Job drawing, mm, ordinate dimensions from the low corner. One solid piece. Coordinates: 2 decimals unless noted, no trailing zeros. Loops run counter-clockwise (first coordinate to the right, second up) from the corner with the lowest first, then second, coordinate; pieces in that order, holes last. Notation, with made-up numbers: (-29.5, -19) - (20.5, -19) arc R29 cw to (20.5, 9) - close; hole circle Ø2 at (76, 85.5). An arc over 180 degrees is marked (long way). Use a Markdown table: item, result. Add a question column.
1. Band-saw the part on A-A, the plane z = 23.5. Give the cut face in (x, y) (1 decimal), plus the area to 3 significant figures.
2. Band-saw the part on C-C, the plane z = 47. Give the cut face in (x, y) (1 decimal).
3. Band-saw the part on B-B, the plane y = 2.45. Count the separate pieces of the cut face and the enclosed holes in it, plus the area to 3 significant figures.
4. Wall check: probe 1 along X at (y, z) = (1.45, 32) (1 decimal); probe 2 along X at (y, z) = (0.55, 47) (1 decimal); probe 3 along Z at (x, y) = (43, 0.5) (1 decimal). Give the ranges that are in metal, low to high. Write a range as [from, to].
5. Drop flat-ended pins along their axis: pin 1 (1 mm diameter, centred on y = 1.5, z = 40, fed in from +X) (1 decimal); pin 2 (1.6 mm diameter, centred on y = 1, z = 36, fed in from -X). Give the stop position or say it passes through.
6. Band-saw the part on D-D, the plane x = 32. Give the cut face in (y, z) (1 decimal).
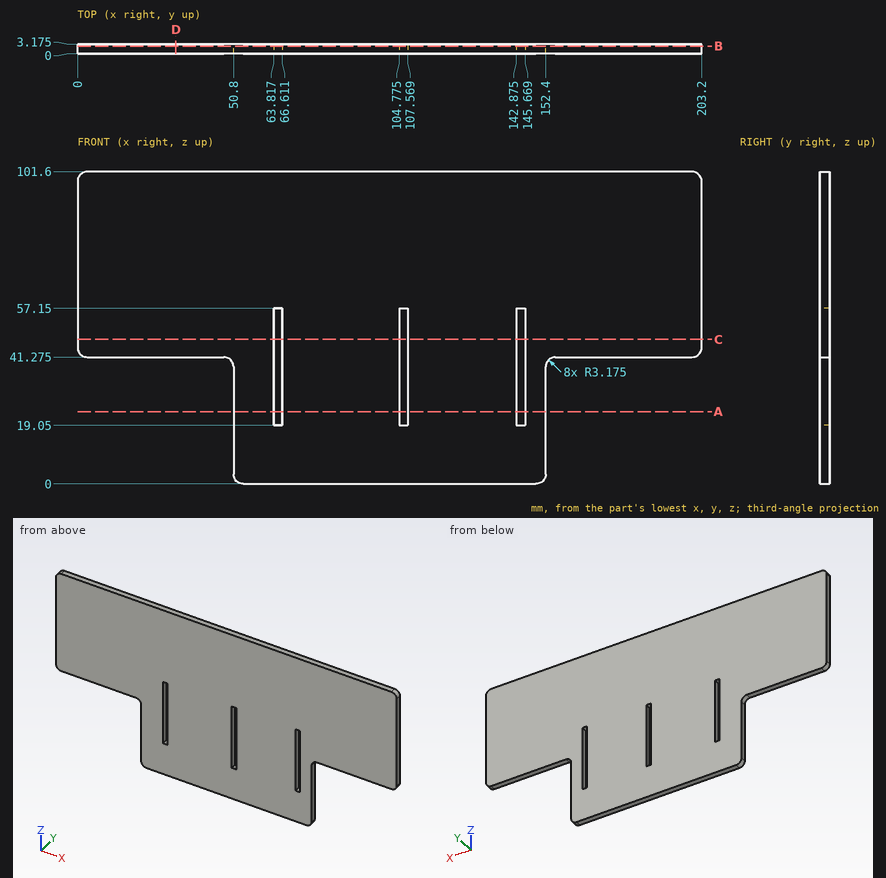
Geometry check:
| question | item | result |
|---|---|---|
| 1 | outline | (50.8, 0) - (63.8, 0) - (63.8, 3.2) - (50.8, 3.2) - close; (66.6, 0) - (104.8, 0) - (104.8, 3.2) - (66.6, 3.2) - close; (107.6, 0) - (142.9, 0) - (142.9, 3.2) - (107.6, 3.2) - close; (145.7, 0) - (152.4, 0) - (152.4, 3.2) - (145.7, 3.2) - close |
| 1 | area | 296 mm^2 |
| 2 | outline | (0, 0) - (63.8, 0) - (63.8, 3.2) - (0, 3.2) - close; (66.6, 0) - (104.8, 0) - (104.8, 3.2) - (66.6, 3.2) - close; (107.6, 0) - (142.9, 0) - (142.9, 3.2) - (107.6, 3.2) - close; (145.7, 0) - (203.2, 0) - (203.2, 3.2) - (145.7, 3.2) - close |
| 3 | separate pieces | 1 |
| 3 | enclosed holes | 3 |
| 3 | area | 16,100 mm^2 |
| 4 | probe 1 | x = [50.8, 63.8], [66.6, 104.8], [107.6, 142.9], [145.7, 152.4] |
| 4 | probe 2 | x = [0, 63.8], [66.6, 104.8], [107.6, 142.9], [145.7, 203.2] |
| 4 | probe 3 | z = [41.3, 101.6] |
| 5 | pin 1 | stops at x = 153.5 |
| 5 | pin 2 | stops at x = 50.8 |
| 6 | outline | (0, 41.3) - (3.2, 41.3) - (3.2, 101.6) - (0, 101.6) - close |
